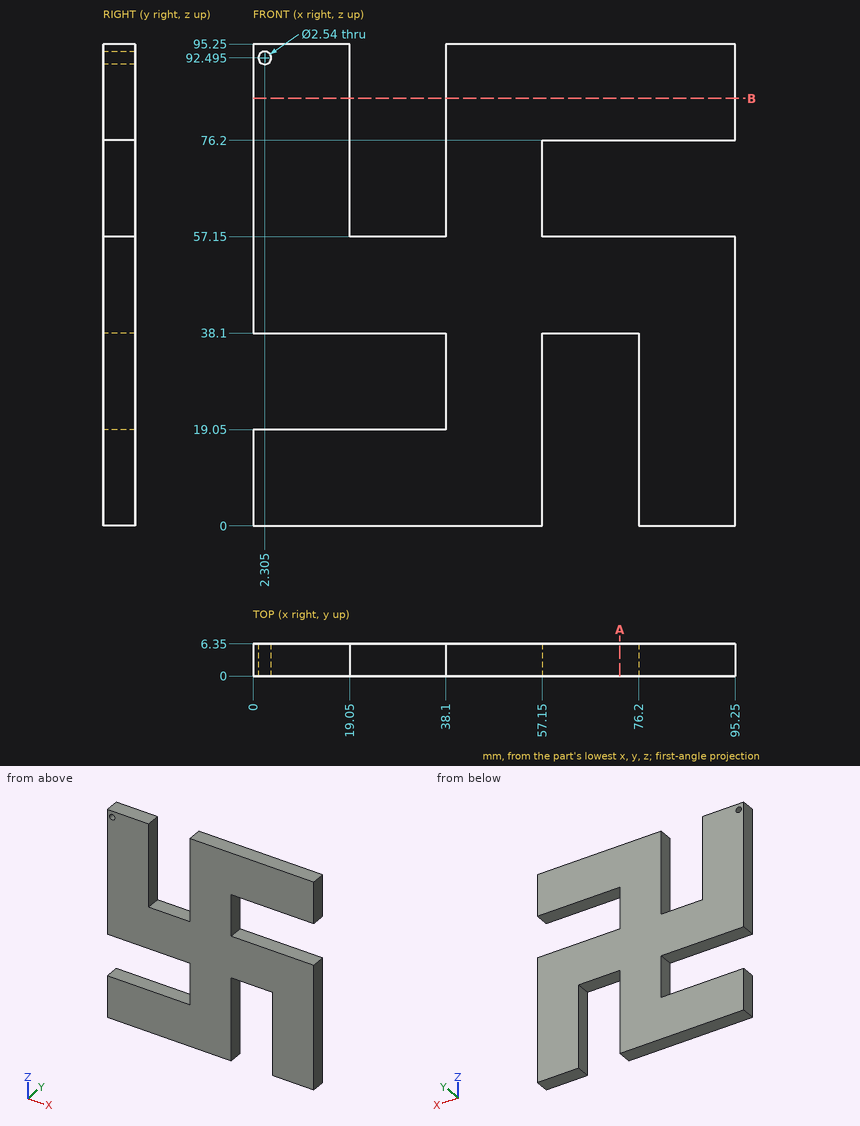
Source: three-view drawing plus pictorial views. Frame: mm from the lowest corner of the part. Give positions to 0.01 mm unless a question says otherwise; leave off trailing zeros. Loops run counter-clockwise (first coordinate to the right, second up) from the corner with the lowest first, then second, coordinate; pieces in that order, holes last.
1) Section query A-A on x = 72.5. Return the cut outline in (y, z), and give its area (3 significant figures).
A:
outline: (0, 38.1) - (6.35, 38.1) - (6.35, 57.15) - (0, 57.15) - close; (0, 76.2) - (6.35, 76.2) - (6.35, 95.25) - (0, 95.25) - close
area: 242 mm2
2) Contact query for flat-ended pins moving along their axis: pin 1 (3 mm diameter, centred on y = 1.5, z = 75, fed in from -X); pin 2 (1.9 mm diameter, centred on y = 3.5, z = 22, fed in from -X); pin 3 (1.9 mm diameter, centred on x = 69, y = 1.5, fed in from -Z); pin 4 (1.9 mm diameter, centred on y = 2.5, z = 63.5, fed in from +X). Output: stop coordinate, or through.
A:
pin 1: stops at x = 0
pin 2: stops at x = 38.1
pin 3: stops at z = 38.1
pin 4: stops at x = 57.15
3) Line query: L1, parallel to X at y = 1.25, z = 85.5; L2, parallel to X at y = 5.75, z = 14. Output: solid intervals per line, ascending.
A:
L1: x = 0 to 19.05, 38.1 to 95.25
L2: x = 0 to 57.15, 76.2 to 95.25
4) Section query B-B on z = 84.5. Return the cut outline in (x, y), and give its area (3 significant figures).
A:
outline: (0, 0) - (19.05, 0) - (19.05, 6.35) - (0, 6.35) - close; (38.1, 0) - (95.25, 0) - (95.25, 6.35) - (38.1, 6.35) - close
area: 484 mm2
